Here's how the part is built. I have some questions about the finished solid (model axes, mm). A direction names the side the tool comes from. Give positions to 0.01 mm unless a question says otherwise; leave off trailing zeros. Loops run counter-clockwise (first coordinate to the right, second up) from the corner with the lowest first, then second, coordinate; pieces in that order, holes last.
Q1. Will these pins go through, and if not, where does the flat tip stop? P1, Ø3.5, axis at x = 75.5, y = 4, coming from the +Z side; P2, Ø3.5, axis at x = 74.5, y = 7, coming from the -Z side.
Q2. We'd pull the mould along Z, two halves only. Please class faces 1 (the face through (75, 5, -15.1)), 2 (the face through (53.2, 5, -12)), 3 (the face through (0, 5, -25)): +Z half, -Z half, draft (parallel to the pull), parting line (faces both ways), or undercut.
Q3. If we section it at B-B (z = -32.5): Please give me the cut outline in (x, y), plus the area to 3 significant figures.
Q4. I need wall thicknesses on line 1 (X direction, y = 3.5, z = -18); line 2 (Z direction, x = 34.5, y = 4.75); line 3 (X direction, y = 6.5, z = -24). Which ranges of each line are inside material? Lowest first, please.
Q5. If we section it at A-A (x = 12): Please give me the cut outline in (y, z).
Q6. For faces 4 (the face through (73.2, 4, -19)), 5 (the face through (75, 5, -35.1)), 6 (the face through (73.2, 6, -31)), 7 (the face through (50.2, 5, -25)), which set-ups out of +Z, -Z, +X, -X, +Y, -Y let a thin tool reach every point of the face, with its end or its side?
Q7. If we section it at C-C (z = -9.5): Please give me the cut outline in (x, y), plus the area to 3 significant figures.
Q8. If we section it at D-D (y = 1.5): Please give me the cut outline in (x, z).
Autodesk Fusion 360 part; units mm, degrees
sketch "Base Mount Sketch" plane through (0, 0, 0) normal (0, 1, 0) x (1, 0, 0) in component "Mount"
  line L0 (0, 0) -> (50.2, 0)
  line L1 (50.2, 0) -> (50.2, 50.2)
  line L2 (50.2, 50.2) -> (0, 50.2)
  line L3 (0, 50.2) -> (0, 0)
  line L4 (73.2, 35.1) -> (76.2, 35.1)
  line L5 (76.2, 35.1) -> (76.2, 15.1)
  line L6 (76.2, 15.1) -> (73.2, 15.1)
  line L7 (73.2, 15.1) -> (73.2, 35.1)
  line L8 (0, 25.1) -> (53.2, 25.1) construction
  line L9 (73.2, 23.6) -> (53.2, 23.6)
  line L10 (53.2, 23.6) -> (53.2, -3)
  line L11 (53.2, -3) -> (-3, -3)
  line L12 (-3, -3) -> (-3, 53.2)
  line L13 (-3, 53.2) -> (53.2, 53.2)
  line L14 (53.2, 53.2) -> (53.2, 26.6)
  line L15 (53.2, 26.6) -> (73.2, 26.6)
  line L16 (53.2, 26.6) -> (53.2, 23.6)
  line L17 (53.2, 25.1) -> (73.2, 25.1) construction
  dimension "d1" = 50.2
  dimension "d2" = 50.2
  dimension "d5" = 3
  dimension "d6" = 20
  dimension "d8" = 3
  dimension "d9" = 3
  dimension "d10" = 3
  dimension "d11" = 3
  dimension "d12" = 3
  dimension "d13" = 20
extrude "Extrude1" add sketch "Base Mount Sketch" along normal blind 10 contours L10 L11 L12 L13 L14 L16 in component "Mount"
sketch "Tweezer Mount Tilt sketch" plane through (53.2, 0, 0) normal (1, 0, 0) x (0, 0, -1) in component "Mount"
  line L0 (-3, 0) -> (53.2, 0)
  line L1 (53.2, 0) -> (53.2, 10)
  line L2 (53.2, 10) -> (-3, 10)
  line L3 (-3, 10) -> (-3, 0)
  line L4 (25.1, 0) -> (25.1, 10) construction
  line L5 (30.2962, 0) -> (24.5226, 10)
  line L6 (25.6774, 0) -> (19.9038, 10)
  line L7 (25.1, 5) -> (30.2962, 0) construction
  line L8 (25.6774, 0) -> (24.5226, 10) construction
  line L9 (19.9038, 10) -> (25.1, 5) construction
  dimension "d25" = 4
  dimension "d32" = 60
extrude "Extrude2" add sketch "Tweezer Mount Tilt sketch" along normal blind 20 contours L0 L2 L5 L6 in component "Mount"
extrude "Extrude3" add sketch "Base Mount Sketch" along normal blind 10 contours L4 L5 L6 L7 in component "Mount"
component "Mount" placed x (1, 0, 0) y (0, 1, 0) z (0, 0, 1) at (0, 0, 0)
equation "d1 = IPA_container_size + fitting_clearance"
equation "d2 = IPA_container_size + fitting_clearance"
equation "nominal_thickness = 3 mm"
equation "IPA_container_size = 50 mm"
equation "d5 = nominal_thickness"
equation "d6 = stopend_width"
equation "d8 = nominal_thickness"
equation "d9 = nominal_thickness"
equation "d10 = nominal_thickness"
equation "d11 = nominal_thickness"
equation "d12 = nominal_thickness"
equation "d13 = tweezer_mount_width"
equation "tweezer_mount_width = 20 mm"
equation "stopend_width = 20 mm"
equation "fitting_clearance = 0.2 mm"
equation "attachment_height = 10 mm"
equation "d18 = attachment_height"
equation "d25 = tweezer_mount_thickness"
equation "tweezer_mount_thickness = nominal_thickness + 1 mm"
equation "d27 = tweezer_mount_width"
equation "d29 = attachment_height"
equation "tweezer_mount_tilt_angle = 60 deg"
equation "d32 = tweezer_mount_tilt_angle"
Check sheet entries:
1. P1: stops at z = -15.1
1. P2: stops at z = -35.1
2. face 1: +Z half
2. face 2: draft
2. face 3: undercut
3. outline: (-3, 0) - (0, 0) - (0, 10) - (-3, 10) - close; (50.2, 0) - (53.2, 0) - (53.2, 10) - (50.2, 10) - close; (73.2, 0) - (76.2, 0) - (76.2, 10) - (73.2, 10) - close
3. area: 90.0 mm2
4. line 1: x = -3 to 0, 50.2 to 53.2, 73.2 to 76.2
4. line 2: z = -53.2 to -50.2, 0 to 3
4. line 3: x = -3 to 0, 50.2 to 76.2
5. outline: (0, -53.2) - (10, -53.2) - (10, -50.2) - (0, -50.2) - close; (0, 0) - (10, 0) - (10, 3) - (0, 3) - close
6. face 4: +Z, -Y
6. face 5: -Z, +X, +Y, -Y
6. face 6: -Z, +Y
6. face 7: +Y, -Y
7. outline: (-3, 0) - (0, 0) - (0, 10) - (-3, 10) - close; (50.2, 0) - (53.2, 0) - (53.2, 10) - (50.2, 10) - close
7. area: 60.0 mm2
8. outline: (-3, -53.2) - (53.2, -53.2) - (53.2, -29.43) - (73.2, -29.43) - (73.2, -35.1) - (76.2, -35.1) - (76.2, -15.1) - (73.2, -15.1) - (73.2, -24.81) - (53.2, -24.81) - (53.2, 3) - (-3, 3) - close; hole (0, -50.2) - (50.2, -50.2) - (50.2, 0) - (0, 0) - close
